```python
from build123d import *

# Parameters (mm, degrees)
SKETCH1_W           = 198
SKETCH1_H           = 111
BOSS_EXTRUDE1_DEPTH = 50.5
SKETCH2_W           = 9.5
SKETCH2_H           = 28
CUT_EXTRUDE1_DEPTH  = 147.5
SKETCH4_R           = 1.5
CUT_EXTRUDE2_DEPTH  = 3


with BuildPart() as part:
    # Sketch1 → Boss-Extrude1 (new body)
    with BuildSketch(Plane(origin=(0, 0, 0), x_dir=(1, 0, 0), z_dir=(0, 1, 0))):
        Rectangle(SKETCH1_W, SKETCH1_H)
    extrude(amount=BOSS_EXTRUDE1_DEPTH)

    # Sketch2 → Cut-Extrude1 (cut)
    with BuildSketch(Plane(origin=(0, 0, -55.5), x_dir=(-1, 0, 0), z_dir=(0, 0, -1))):
        with Locations((94.25, 36.5)):
            Rectangle(SKETCH2_W, SKETCH2_H)
    extrude(amount=-CUT_EXTRUDE1_DEPTH, mode=Mode.SUBTRACT)

    # Sketch4 → Cut-Extrude2 (cut)
    with BuildSketch(Plane.XZ):
        with Locations((87, 39.5)):
            Circle(SKETCH4_R)
        with Locations((87, -45.5)):
            Circle(SKETCH4_R)
        with Locations((-39, 39.5)):
            Circle(SKETCH4_R)
        with Locations((-39, -45.5)):
            Circle(SKETCH4_R)
    extrude(amount=-CUT_EXTRUDE2_DEPTH, mode=Mode.SUBTRACT)


solid = part.part
```
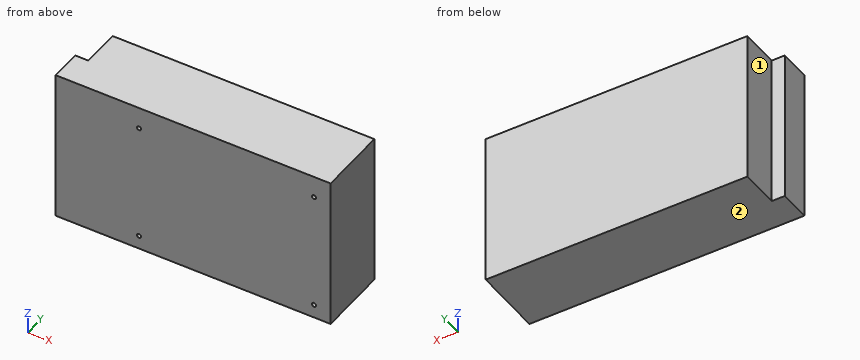
CAD build for the part. Positions are in the model's coordinates, mm. Face numbers are marked on the shaded views. A direction names the side the tool comes from. Round coordinates to 2 decimals unless told otherwise and drop trailing zeros. Loops run counter-clockwise (first coordinate to the right, second up) from the corner with the lowest first, then second, coordinate; pieces in that order, holes last. Notation, with made-up numbers: (5.5, 77.25) - (57.5, 77.25) arc R25 cw to (57.5, 93.25) - close; hole circle Ø2 at (35, 76.25). An arc over 180 degrees is marked (long way). Return JSON: item names as keys, results as strings. Group by question number.
Q1. Tool access for the marked faces 1 and 2: list every direction of +Z, -Z, +X, -X, +Y, -Y with a clear straight run to the whole face (end or side of a thin tool).
Q2. Band-saw the part on A-A on z = -24. Give the cut face in (x, y), plus the area to 3 significant figures.
Q3. Flat gauge pin, fed straight in: pin 1 Ø2.5 at (x, z) = (87, 39.5) entering from -Y. Where does the tip first touch, or does it go through?
Q4. Band-saw the part on B-B on y = 32. Give the cut face in (x, z).
Q5. Drill centre lines: line 1 along Z through (x, y) = (-39, 2); line 2 along X through (y, z) = (1, -45); line 3 along X through (y, z) = (37.5, -7). Where is each one in solid material? Low to high. Write a range as [from, to].
Solutions:
{
 "1": {"face 1": "+Z, -Z, -X, +Y", "face 2": "-Z, +X, -X, +Y, -Y"},
 "2": {"outline": "(-99, 0) - (99, 0) - (99, 50.5) - (-89.5, 50.5) - (-89.5, 22.5) - (-99, 22.5) - close", "area": "9,730 mm^2"},
 "3": {"pin 1": "stops at y = 3"},
 "4": {"outline": "(-89.5, -55.5) - (99, -55.5) - (99, 55.5) - (-89.5, 55.5) - close"},
 "5": {"line 1": "z = [-55.5, -47], [-44, 38], [41, 55.5]", "line 2": "x = [-99, -40.41], [-37.59, 85.59], [88.41, 99]", "line 3": "x = [-89.5, 99]"}
}
